from build123d import *

# Parameters (mm, degrees)
F0_R     = 11.5
F0_W     = 20
F0_H     = 20
F0_R_2   = 3
F0_R_3   = 10.9
F1_DEPTH = 2
F2_R     = 3


with BuildPart() as f1:
    # F0 (on Top) → F1 (new body)
    with BuildSketch(Plane.XY):
        Polygon((25, 17.5), (-25, 17.5), (-25, 10), (-25, -10), (-25, -17.5), (25, -17.5), (25, -10), (25, 10), align=None)
        Circle(F0_R, mode=Mode.SUBTRACT)
        with Locations((-35, 0)):
            Rectangle(F0_W, F0_H)
        with Locations((-35, 0)):
            Circle(F0_R_2, mode=Mode.SUBTRACT)
        with Locations((35, 0)):
            Rectangle(F0_W, F0_H)
        with Locations((35, 0)):
            Circle(F0_R_2, mode=Mode.SUBTRACT)
        Circle(F0_R)
        Circle(F0_R_3, mode=Mode.SUBTRACT)
    extrude(amount=F1_DEPTH)

    # F2
    f2_edges = [f1.edges().sort_by_distance(p)[0] for p in [
        (-25, -10, 1),
        (-25, 10, 1),
        (25, 10, 1),
        (25, -10, 1),
        (25, 17.5, 1),
        (25, -17.5, 1),
        (-25, -17.5, 1),
        (-25, 17.5, 1),
        (-45, 10, 1),
        (-45, -10, 1),
        (45, -10, 1),
        (45, 10, 1),
    ]]
    fillet(f2_edges, radius=F2_R)


solid = f1.part
The model under review builds one solid part; all positions refer to its coordinate system, in mm. A direction names the side the tool comes from. Round coordinates to 2 decimals unless told otherwise and drop trailing zeros. Loops run counter-clockwise (first coordinate to the right, second up) from the corner with the lowest first, then second, coordinate; pieces in that order, holes last. Notation, with made-up numbers: M 48,-24.75 L 89,-24.75 A26 ccw 89,14.25 Z; hole C 35.25,-16.5 d4. An arc over 180 degrees is marked long. Answer as a JSON object with one key per item and string values.
Item 1: We need section B-B, the plane z = 0.65. State the section outline as (x, y) points.
Check sheet entries:
{"outline": "M -45,-7 A3 ccw -42,-10 L -28,-10 A3 cw -25,-13 L -25,-14.5 A3 ccw -22,-17.5 L 22,-17.5 A3 ccw 25,-14.5 L 25,-13 A3 cw 28,-10 L 42,-10 A3 ccw 45,-7 L 45,7 A3 ccw 42,10 L 28,10 A3 cw 25,13 L 25,14.5 A3 ccw 22,17.5 L -22,17.5 A3 ccw -25,14.5 L -25,13 A3 cw -28,10 L -42,10 A3 ccw -45,7 Z; hole C -35,0 d6; hole C 0,0 d21.8; hole C 35,0 d6"}
Item 2: The part is to be moulded in two halves that separate along Y. For faces 1 (the face through (-35, -10, 1)), 2 (the face through (35, 10, 1)), 3 (the face through (10.4, 3.27, 0.99)), say which applies: +Y half, -Y half, draft (parallel to the pull), parting line (faces both ways), or undercut.
Check sheet entries:
{"face 1": "-Y half", "face 2": "+Y half", "face 3": "undercut"}
Item 3: Tool access review of faces 4 (the face through (25, -14, 1)), 5 (the face through (-25.9, -10.86, 1.01)), 6 (the face through (-25, 14, 1)): name each direction out of +Z, -Z, +X, -X, +Y, -Y from which nothing blocks a thin tool from reaching the whole face with its end or side.
Check sheet entries:
{"face 4": "+Z, -Z, +X, -Y", "face 5": "+Z, -Z, -X, -Y", "face 6": "+Z, -Z, -X, +Y"}
Item 4: We need section C-C, the plane x = -35. State the section outline as (y, z) points, and give its area (3 significant figures).
Check sheet entries:
{"outline": "M -10,0 L -3,0 L -3,2 L -10,2 Z; M 3,0 L 10,0 L 10,2 L 3,2 Z", "area": "28.0 mm2"}
Item 5: We need section A-A, the plane y = 0. State the section outline as (x, z) points.
Check sheet entries:
{"outline": "M -45,0 L -38,0 L -38,2 L -45,2 Z; M -32,0 L -10.9,0 L -10.9,2 L -32,2 Z; M 10.9,0 L 32,0 L 32,2 L 10.9,2 Z; M 38,0 L 45,0 L 45,2 L 38,2 Z"}
Item 6: We need section D-D, the plane x = 39. State the section outline as (y, z) points.
Check sheet entries:
{"outline": "M -10,0 L 10,0 L 10,2 L -10,2 Z"}
Item 7: Clearance check with flat-ended pins moving along their axes: P1, Ø0.8, axis at y = -14, z = 1, coming from the -X side; P2, Ø0.6, axis at x = -36, z = 0.5, coming from the -Y side; P3, Ø1.2, axis at y = 14, z = 0.5, coming from the +X side. State where each tip first meets the part, or that it passes through.
Check sheet entries:
{"P1": "x = -25", "P2": "y = -10", "P3": "x = 25"}
Item 8: For line 1 along Y through (x, z) = (35, 0.9); line 2 along X through (y, z) = (-0.5, 0.95); line 3 along Y through (x, z) = (-37.5, 0.4), list the stretches that pass through material, from the lowest coordinate up.
Check sheet entries:
{"line 1": "-10 to -3, 3 to 10", "line 2": "-45 to -37.96, -32.04 to -10.89, 10.89 to 32.04, 37.96 to 45", "line 3": "-10 to -1.66, 1.66 to 10"}
